```python
from build123d import *

# Parameters (mm, degrees)
SKETCH1_W                        = 1171.575
SKETCH1_H                        = 571.5
BOSS_EXTRUDE1_DEPTH              = 6.35
F_27_64_0_42188_DIAMETER_HOLE1_D = 10.715752
SKETCH5_W                        = 44.45
SKETCH5_H                        = 76.2
CUT_EXTRUDE1_DEPTH               = 7.35
CUT_EXTRUDE2_DEPTH               = 7.35
FILLET1_R                        = 12.7
FILLET2_R                        = 2.54


with BuildPart() as part:
    # Sketch1 → Boss-Extrude1 (new body)
    with BuildSketch(Plane.XY):
        with Locations((0, 285.75)):
            Rectangle(SKETCH1_W, SKETCH1_H)
    extrude(amount=BOSS_EXTRUDE1_DEPTH)

    # 27/64 (0.42188) Diameter Hole1 (through all)
    with Locations(Plane.XY.offset(6.35)):
        with Locations((304.8, 495.3), (-247.65, 495.3), (-304.8, 495.3), (-247.65, 76.2), (-304.8, 76.2), (247.65, 76.2), (304.8, 76.2), (247.65, 495.3)):
            Hole(F_27_64_0_42188_DIAMETER_HOLE1_D / 2)

    # Sketch5 → Cut-Extrude1 (cut, through all)
    with BuildSketch(Plane.XY.offset(6.35)):
        with Locations((-476.25, 533.4)):
            Rectangle(SKETCH5_W, SKETCH5_H)
        with Locations((0, 533.4)):
            Rectangle(SKETCH5_W, SKETCH5_H)
        with Locations((476.25, 533.4)):
            Rectangle(SKETCH5_W, SKETCH5_H)
    extrude(amount=-CUT_EXTRUDE1_DEPTH, mode=Mode.SUBTRACT)

    # Sketch6 → Cut-Extrude2 (cut, through all)
    with BuildSketch(Plane.XY.offset(6.35)):
        with BuildLine():
            Line((4.7625, 0), (-4.7625, 0))
            Line((-4.7625, 0), (-4.7625, 11.1125))
            ThreePointArc((-4.7625, 11.1125), (0, 15.875), (4.7625, 11.1125))
            Line((4.7625, 11.1125), (4.7625, 0))
        make_face()
    extrude(amount=-CUT_EXTRUDE2_DEPTH, mode=Mode.SUBTRACT)

    # Fillet1
    fillet1_edges = [part.edges().sort_by_distance(p)[0] for p in [
        (-454.025, 495.3, 3.175),
        (-498.475, 495.3, 3.175),
        (-22.225, 495.3, 3.175),
        (22.225, 495.3, 3.175),
        (454.025, 495.3, 3.175),
        (498.475, 495.3, 3.175),
    ]]
    fillet(fillet1_edges, radius=FILLET1_R)

    # Fillet2
    fillet2_edges = [part.edges().sort_by_distance(p)[0] for p in [
        (4.7625, 0, 3.175),
        (-4.7625, 0, 3.175),
        (-498.475, 571.5, 3.175),
        (-454.025, 571.5, 3.175),
        (-585.7875, 571.5, 3.175),
        (585.7875, 571.5, 3.175),
        (585.7875, 0, 3.175),
        (-22.225, 571.5, 3.175),
        (-585.7875, 0, 3.175),
        (22.225, 571.5, 3.175),
        (454.025, 571.5, 3.175),
        (498.475, 571.5, 3.175),
    ]]
    fillet(fillet2_edges, radius=FILLET2_R)


solid = part.part
```
Design review of the part built by this model. Coordinates are the model's own, in mm. Give positions to 0.01 mm unless a question says otherwise; leave off trailing zeros. Return JSON: item names as keys, results as strings. Group by question number.
Item 1: For probe 1 along X at (y, z) = (520, 4.75) (1 decimal); probe 2 along Y at (x, z) = (304.5, 3.25); probe 3 along Y at (x, z) = (-249, 3.5), list the stretches that pass through material, from the lowest coordinate up.
Item 2: Insertion check: pin 1 Ø9.5 at (x, y) = (304.8, 76.2) entering from +Z; pin 2 Ø3 at (x, z) = (3.5, 3) entering from +Y. Each pin has a flat end and moves straight along its axis. Give the tip position at first contact, or say it passes through.
Item 3: We need section A-A (z = 2.5). Give the number of separate pieces and of enclosed holes in the cut face, and give its area (3 significant figures).
Output:
{
 "1": {"probe 1": "x = -585.8 to -498.5, -454 to -22.2, 22.2 to 454, 498.5 to 585.8", "probe 2": "y = 0 to 70.85, 81.55 to 489.95, 500.65 to 571.5", "probe 3": "y = 0 to 71.01, 81.39 to 490.11, 500.49 to 571.5"},
 "2": {"pin 1": "passes through", "pin 2": "stops at y = 495.3"},
 "3": {"separate pieces": "1", "enclosed holes": "8", "area": "659,000 mm^2"}
}
